Part model, mm, in its own coordinate system. A direction names the side the tool comes from. Give positions to 0.01 mm unless a question says otherwise; leave off trailing zeros. Write each loop counter-clockwise with the first axis right and the second up, starting at its lowest first coordinate (ties: lowest second). Pieces come first, ordered by that corner, then holes.
from build123d import *

# Parameters (mm, degrees)
SKETCH1_R           = 2.5
BOSS_EXTRUDE1_DEPTH = 16
SKETCH2_R           = 4
BOSS_EXTRUDE2_DEPTH = 3
FILLET1_R           = 1


with BuildPart() as part:
    # Sketch1 → Boss-Extrude1 (new body)
    with BuildSketch(Plane.XY):
        with Locations((-20, -30)):
            Circle(SKETCH1_R)
    extrude(amount=-BOSS_EXTRUDE1_DEPTH)

    # Sketch2 → Boss-Extrude2 (add)
    with BuildSketch(Plane.XY):
        with Locations((-20, -30)):
            Circle(SKETCH2_R)
    extrude(amount=BOSS_EXTRUDE2_DEPTH)

    # Fillet1
    fillet1_edges = [part.edges().sort_by_distance(p)[0] for p in [
        (-24, -30, 3),
    ]]
    fillet(fillet1_edges, radius=FILLET1_R)


solid = part.part
1) Flat gauge pins, fed straight in: P1, Ø3, axis at x = -17.5, z = -8, coming from the +Y side; P2, Ø2, axis at x = -18.5, z = -7.5, coming from the -Y side. Where does each tip first touch, or does it go through?
Check result:
P1: stops at y = -27.71
P2: stops at y = -32.45
2) Saw through at C-C (z = -9). Write the cut outline in (x, y).
Check result:
outline: circle Ø5 at (-20, -30)
3) 3-axis set-ups, long thin cutter, end or side, ignore diameter. For faces 1 (the flat face through (-18, -28, 0)), 2 (the flat face through (-20, -30, 3)): which of +Z, -Z, +X, -X, +Y, -Y reach the whole face in a straight line?
Check result:
face 1: -Z
face 2: +Z, +X, -X, +Y, -Y
4) Saw through at A-A (x = -20). Write the cut outline in (y, z), and give its area (3 significant figures).
Check result:
outline: (-34, 0) - (-32.5, 0) - (-32.5, -16) - (-27.5, -16) - (-27.5, 0) - (-26, 0) - (-26, 2) arc R1 ccw to (-27, 3) - (-33, 3) arc R1 ccw to (-34, 2) - close
area: 104 mm2
5) Saw through at B-B (y = -30). Write the cut outline in (x, z), and give its area (3 significant figures).
Check result:
outline: (-24, 0) - (-22.5, 0) - (-22.5, -16) - (-17.5, -16) - (-17.5, 0) - (-16, 0) - (-16, 2) arc R1 ccw to (-17, 3) - (-23, 3) arc R1 ccw to (-24, 2) - close
area: 104 mm2
6) Drill centre lines: L1, parallel to Z at x = -17, y = -29.25; L2, parallel to X at y = -32, z = -10; L3, parallel to X at y = -30.75, z = -11.5. Where is each one in solid material? Low to high.
Check result:
L1: z = 0 to 3
L2: x = -21.5 to -18.5
L3: x = -22.38 to -17.62
